Input: part model. Units: mm. Frame: model coordinates. Round coordinates to 2 decimals unless told otherwise and drop trailing zeros. Write each loop counter-clockwise with the first axis right and the second up, starting at its lowest first coordinate (ties: lowest second). Pieces come first, ordered by that corner, then holes. Notation, with made-up numbers: (29.25, -10) -> (80.25, -10) arc R25 cw to (80.25, 4) -> close; hole circle Ø6 at (34.5, 42). An arc over 180 degrees is marked (long way). Write item = value, one per line.
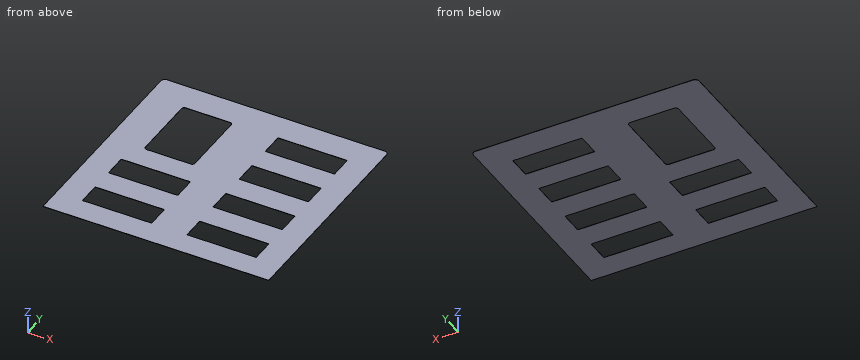
```python
from build123d import *

# Parameters (mm, degrees)
BASE_FLANGE1_DEPTH = 1
CUT_EXTRUDE1_DEPTH = 10
CUT_EXTRUDE2_DEPTH = 10


# Sheet-metal steps are written as plain solids
with BuildPart() as part:
    # Sketch1 → Base-Flange1 (new body)
    with BuildSketch(Plane.XY):
        with BuildLine():
            Line((0, 0), (863.4, 0))
            Line((863.4, 0), (863.4, 812))
            ThreePointArc((863.4, 812), (858.801576465, 823.101576465), (847.7, 827.7))
            Line((847.7, 827.7), (15.7, 827.7))
            ThreePointArc((15.7, 827.7), (4.598423535, 823.101576465), (0, 812))
            Line((0, 812), (0, 0))
        make_face()
    extrude(amount=-BASE_FLANGE1_DEPTH)

    # Sketch9 → Cut-Extrude1 (cut)
    with BuildSketch(Plane.XY):
        with BuildLine():
            Line((762.2, 720.7), (501.2, 720.7))
            ThreePointArc((501.2, 720.7), (499.785786438, 720.114213562), (499.2, 718.7))
            Line((499.2, 718.7), (499.2, 634.7))
            ThreePointArc((499.2, 634.7), (499.785786438, 633.285786438), (501.2, 632.7))
            Line((501.2, 632.7), (762.2, 632.7))
            ThreePointArc((762.2, 632.7), (763.614213562, 633.285786438), (764.2, 634.7))
            Line((764.2, 634.7), (764.2, 718.7))
            ThreePointArc((764.2, 718.7), (763.614213562, 720.114213562), (762.2, 720.7))
        make_face()
        with BuildLine():
            Line((764.2, 538.7), (764.2, 454.7))
            ThreePointArc((764.2, 454.7), (763.614213562, 453.285786438), (762.2, 452.7))
            Line((762.2, 452.7), (501.2, 452.7))
            ThreePointArc((501.2, 452.7), (499.785786438, 453.285786438), (499.2, 454.7))
            Line((499.2, 454.7), (499.2, 538.7))
            ThreePointArc((499.2, 538.7), (499.785786438, 540.114213562), (501.2, 540.7))
            Line((501.2, 540.7), (762.2, 540.7))
            ThreePointArc((762.2, 540.7), (763.614213562, 540.114213562), (764.2, 538.7))
        make_face()
        with BuildLine():
            Line((764.2, 358.7), (764.2, 274.7))
            ThreePointArc((764.2, 274.7), (763.614213562, 273.285786438), (762.2, 272.7))
            Line((762.2, 272.7), (501.2, 272.7))
            ThreePointArc((501.2, 272.7), (499.785786438, 273.285786438), (499.2, 274.7))
            Line((499.2, 274.7), (499.2, 358.7))
            ThreePointArc((499.2, 358.7), (499.785786438, 360.114213562), (501.2, 360.7))
            Line((501.2, 360.7), (762.2, 360.7))
            ThreePointArc((762.2, 360.7), (763.614213562, 360.114213562), (764.2, 358.7))
        make_face()
        with BuildLine():
            Line((764.2, 178.7), (764.2, 94.7))
            ThreePointArc((764.2, 94.7), (763.614213562, 93.285786438), (762.2, 92.7))
            Line((762.2, 92.7), (501.2, 92.7))
            ThreePointArc((501.2, 92.7), (499.785786438, 93.285786438), (499.2, 94.7))
            Line((499.2, 94.7), (499.2, 178.7))
            ThreePointArc((499.2, 178.7), (499.785786438, 180.114213562), (501.2, 180.7))
            Line((501.2, 180.7), (762.2, 180.7))
            ThreePointArc((762.2, 180.7), (763.614213562, 180.114213562), (764.2, 178.7))
        make_face()
        with BuildLine():
            Line((364.2, 358.7), (364.2, 274.7))
            ThreePointArc((364.2, 274.7), (363.614213562, 273.285786438), (362.2, 272.7))
            Line((362.2, 272.7), (101.2, 272.7))
            ThreePointArc((101.2, 272.7), (99.785786438, 273.285786438), (99.2, 274.7))
            Line((99.2, 274.7), (99.2, 358.7))
            ThreePointArc((99.2, 358.7), (99.785786438, 360.114213562), (101.2, 360.7))
            Line((101.2, 360.7), (362.2, 360.7))
            ThreePointArc((362.2, 360.7), (363.614213562, 360.114213562), (364.2, 358.7))
        make_face()
        with BuildLine():
            Line((364.2, 178.7), (364.2, 94.7))
            ThreePointArc((364.2, 94.7), (363.614213562, 93.285786438), (362.2, 92.7))
            Line((362.2, 92.7), (101.2, 92.7))
            ThreePointArc((101.2, 92.7), (99.785786438, 93.285786438), (99.2, 94.7))
            Line((99.2, 94.7), (99.2, 178.7))
            ThreePointArc((99.2, 178.7), (99.785786438, 180.114213562), (101.2, 180.7))
            Line((101.2, 180.7), (362.2, 180.7))
            ThreePointArc((362.2, 180.7), (363.614213562, 180.114213562), (364.2, 178.7))
        make_face()
    extrude(amount=-CUT_EXTRUDE1_DEPTH, mode=Mode.SUBTRACT)

    # Sketch10 → Cut-Extrude2 (cut)
    with BuildSketch(Plane.XY):
        with BuildLine():
            Line((146.7, 449.2), (316.7, 449.2))
            ThreePointArc((316.7, 449.2), (323.771067812, 452.128932188), (326.7, 459.2))
            Line((326.7, 459.2), (326.7, 709.2))
            ThreePointArc((326.7, 709.2), (323.771067812, 716.271067812), (316.7, 719.2))
            Line((316.7, 719.2), (146.7, 719.2))
            ThreePointArc((146.7, 719.2), (139.628932188, 716.271067812), (136.7, 709.2))
            Line((136.7, 709.2), (136.7, 459.2))
            ThreePointArc((136.7, 459.2), (139.628932188, 452.128932188), (146.7, 449.2))
        make_face()
    extrude(amount=-CUT_EXTRUDE2_DEPTH, mode=Mode.SUBTRACT)


solid = part.part
```
1) Cut plane D-D (z = -0.4). Count the separate pieces of the cut face and the enclosed holes in it, and give its area (3 significant figures).
Solutions:
separate_pieces = 1
enclosed_holes = 7
area = 523,000 mm^2
2) Line query: L1, parallel to X at y = 284.5, z = -0.5; L2, parallel to X at y = 675, z = -0.2; L3, parallel to Y at x = 569, z = -0.35. Output: solid intervals per line, ascending. Write a range as from..to.
Solutions:
L1 = 0..99.2, 364.2..499.2, 764.2..863.4
L2 = 0..136.7, 326.7..499.2, 764.2..863.4
L3 = 0..92.7, 180.7..272.7, 360.7..452.7, 540.7..632.7, 720.7..827.7
3) First-contact query: P1, Ø10, axis at x = 501, y = 221.5, coming from the +Z side. Flat tip, straight axial feed; report the tip coordinate or a pass-through.
Solutions:
P1 = 0
4) Cut plane A-A (y = 667). Return the cut outline in (x, z), and give its area (3 significant figures).
Solutions:
outline = (0, -1) -> (136.7, -1) -> (136.7, 0) -> (0, 0) -> close; (326.7, -1) -> (499.2, -1) -> (499.2, 0) -> (326.7, 0) -> close; (764.2, -1) -> (863.4, -1) -> (863.4, 0) -> (764.2, 0) -> close
area = 408 mm^2
5) Cut plane C-C (x = 561.5). Return the cut outline in (y, z).
Solutions:
outline = (0, -1) -> (92.7, -1) -> (92.7, 0) -> (0, 0) -> close; (180.7, -1) -> (272.7, -1) -> (272.7, 0) -> (180.7, 0) -> close; (360.7, -1) -> (452.7, -1) -> (452.7, 0) -> (360.7, 0) -> close; (540.7, -1) -> (632.7, -1) -> (632.7, 0) -> (540.7, 0) -> close; (720.7, -1) -> (827.7, -1) -> (827.7, 0) -> (720.7, 0) -> close
6) Cut plane B-B (y = 560). Return the cut outline in (x, z), and give its area (3 significant figures).
Solutions:
outline = (0, -1) -> (136.7, -1) -> (136.7, 0) -> (0, 0) -> close; (326.7, -1) -> (863.4, -1) -> (863.4, 0) -> (326.7, 0) -> close
area = 673 mm^2
